Part model, mm, in its own coordinate system. Face numbers are marked on the shaded views. A direction names the side the tool comes from. Round coordinates to 2 decimals unless told otherwise and drop trailing zeros. Loops run counter-clockwise (first coordinate to the right, second up) from the corner with the lowest first, then second, coordinate; pieces in that order, holes last.
(1) Probe probe 1 along Z at (x, y) = (40.5, -22) (3 decimals); probe 2 along X at (y, z) = (-87.5, 5) (3 decimals); probe 3 along Z at (x, y) = (76.5, -57) (3 decimals). List the from-to ranges inside material, lowest first.
(2) Cut at B-B on x = 84.5. List the corners of the cut face in (y, z) (3 decimals).
(3) Tool access for the marked faces 1 and 2: list every direction of +Z, -Z, +X, -X, +Y, -Y with a clear straight run to the whole face (end or side of a thin tool).
(4) Mould opens along X. For the marked faces 3, 4, 5 and 6 say: +X half, -X half, draft (parallel to the pull), parting line (faces both ways), or undercut.
(5) Cut at A-A on z = -1.5. List the corners of the cut face in (x, y) (3 decimals).
(6) Flat gauge pins, fed straight in: pin 1 (1.5 mm diameter, centred on x = 65.5, y = -74, fed in from -Z); pin 2 (2 mm diameter, centred on x = -10, y = -90.5, fed in from +Z); pin 3 (1.6 mm diameter, centred on x = 59, y = -94, fed in from -Z). Where does each tip first touch, or does it go through?
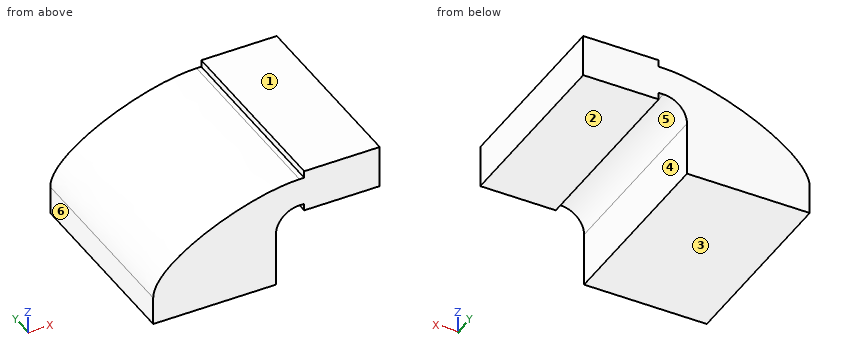
from build123d import *

# Parameters (mm, degrees)
F0_W     = 82.55
F0_H     = 19.05
F0_W_2   = 27.7625424093
F0_H_2   = 4.7498
F0_H_3   = 4.7752
F1_DEPTH = 127


with BuildPart() as f1:
    # F0 (on Front) → F1 (new body)
    with BuildSketch(Plane.XZ):
        with BuildLine():
            add(Edge.make_bspline(
                [(-41.275, 9.525), (-41.275, 33.9924029201), (21.7312667782, 61.9252), (57.15, 61.9252)],
                knots=[0, 0, 0, 0, 111.5045361635, 111.5045361635, 111.5045361635, 111.5045361635], degree=3))
            Line((-41.275, 9.525), (41.275, 9.525))
            Line((41.275, 9.525), (41.275, 27.0002))
            ThreePointArc((41.275, 27.0002), (45.9246798487, 38.2255201513), (57.15, 42.8752))
            Line((57.15, 42.8752), (60.325, 42.8752))
            Line((60.325, 42.8752), (60.325, 61.9252))
            Line((60.325, 61.9252), (57.15, 61.9252))
        make_face()
        Rectangle(F0_W, F0_H)
        with Locations((74.2062712047, 52.4002)):
            Rectangle(F0_W_2, F0_H)
        with Locations((74.2062712047, 64.3001)):
            Rectangle(F0_W_2, F0_H_2)
        with Locations((74.2062712047, 40.4876)):
            Rectangle(F0_W_2, F0_H_3)
        Polygon((88.0875424093, 66.675), (88.0875424093, 61.9252), (88.0875424093, 42.8752), (88.0875424093, 38.1), (111.125, 38.1), (111.125, 66.675), align=None)
    extrude(amount=F1_DEPTH)


solid = f1.part
Final values:
1. probe 1: z = -9.525 to 60.298
1. probe 2: x = -41.275 to 41.275
1. probe 3: z = 38.1 to 66.675
2. outline: (-127, 38.1) - (0, 38.1) - (0, 66.675) - (-127, 66.675) - close
3. face 1: +Z, +X, -X, +Y, -Y
3. face 2: -Z, +X, +Y, -Y
4. face 3: draft
4. face 4: +X half
4. face 5: undercut
4. face 6: -X half
5. outline: (-41.275, -127) - (41.275, -127) - (41.275, 0) - (-41.275, 0) - close
6. pin 1: stops at z = 38.1
6. pin 2: stops at z = 43.02
6. pin 3: stops at z = 42.88
